from build123d import *

# Parameters (mm, degrees)
SKETCH1_R           = 1.450000001
SKETCH1_R_2         = 3.250000001
SKETCH1_R_3         = 1.5
SKETCH1_R_4         = 2.5
SKETCH1_R_5         = 1.375000001
BOSS_EXTRUDE2_DEPTH = 6.35


with BuildPart() as part:
    # Sketch1 → Boss-Extrude2 (new body)
    with BuildSketch(Plane.XY):
        with BuildLine():
            Line((-155.352886895, 10.211716756), (-51.913748531, 10.211716756))
            ThreePointArc((-51.913748531, 10.211716756), (-39.74822347, 6.086224622), (-32.601576204, -4.588283244))
            ThreePointArc((-32.601576204, -4.588283244), (53.610301025, -63.284580406), (124.587919611, 13.13479368))
            ThreePointArc((124.587919611, 13.13479368), (56.661218885, 95.304455124), (-32.601576204, 37.011716756))
            ThreePointArc((-32.601576204, 37.011716756), (-39.74822347, 26.33720889), (-51.913748531, 22.211716756))
            Line((-51.913748531, 22.211716756), (-155.352886895, 22.211716756))
            ThreePointArc((-155.352886895, 22.211716756), (-161.352886895, 16.211716756), (-155.352886895, 10.211716756))
        make_face()
        with Locations((-19.438766774, -20.788283242)):
            Circle(SKETCH1_R, mode=Mode.SUBTRACT)
        with Locations((-26.831398039, -2.940892579)):
            Circle(SKETCH1_R, mode=Mode.SUBTRACT)
        with Locations((-155.352886895, 16.211716756)):
            Circle(SKETCH1_R_2, mode=Mode.SUBTRACT)
        with Locations((-26.831398039, 35.364326096)):
            Circle(SKETCH1_R, mode=Mode.SUBTRACT)
        with Locations((-19.438766774, 53.211716759)):
            Circle(SKETCH1_R, mode=Mode.SUBTRACT)
        with Locations((-29.352886893, 16.211716758)):
            Circle(SKETCH1_R, mode=Mode.SUBTRACT)
        with Locations((44.647113106, 6.211716759)):
            Circle(SKETCH1_R_3, mode=Mode.SUBTRACT)
        with Locations((116.125624253, -2.940892579)):
            Circle(SKETCH1_R, mode=Mode.SUBTRACT)
        with Locations((108.732992988, -20.788283242)):
            Circle(SKETCH1_R, mode=Mode.SUBTRACT)
        with Locations((96.973014915, -36.114185049)):
            Circle(SKETCH1_R, mode=Mode.SUBTRACT)
        with Locations((81.647113106, -47.874163121)):
            Circle(SKETCH1_R, mode=Mode.SUBTRACT)
        with Locations((63.799722443, -55.266794386)):
            Circle(SKETCH1_R, mode=Mode.SUBTRACT)
        with Locations((44.647113106, -57.788283242)):
            Circle(SKETCH1_R, mode=Mode.SUBTRACT)
        with Locations((25.494503768, -55.266794386)):
            Circle(SKETCH1_R, mode=Mode.SUBTRACT)
        with Locations((7.647113108, -47.874163121)):
            Circle(SKETCH1_R, mode=Mode.SUBTRACT)
        with Locations((-7.678788702, -36.114185049)):
            Circle(SKETCH1_R, mode=Mode.SUBTRACT)
        with Locations((44.647113106, 16.211716756)):
            Circle(SKETCH1_R_4, mode=Mode.SUBTRACT)
        with Locations((-7.678788702, 68.537618566)):
            Circle(SKETCH1_R, mode=Mode.SUBTRACT)
        with Locations((7.647113108, 80.297596638)):
            Circle(SKETCH1_R, mode=Mode.SUBTRACT)
        with Locations((25.494503768, 87.690227903)):
            Circle(SKETCH1_R, mode=Mode.SUBTRACT)
        with Locations((44.647113106, 90.211716759)):
            Circle(SKETCH1_R, mode=Mode.SUBTRACT)
        with Locations((63.799722443, 87.690227903)):
            Circle(SKETCH1_R, mode=Mode.SUBTRACT)
        with Locations((81.647113106, 80.297596638)):
            Circle(SKETCH1_R, mode=Mode.SUBTRACT)
        with Locations((96.973014915, 68.537618566)):
            Circle(SKETCH1_R, mode=Mode.SUBTRACT)
        with Locations((108.732992988, 53.211716759)):
            Circle(SKETCH1_R, mode=Mode.SUBTRACT)
        with Locations((116.125624253, 35.364326096)):
            Circle(SKETCH1_R, mode=Mode.SUBTRACT)
        with Locations((44.647113106, 26.211716758)):
            Circle(SKETCH1_R_5, mode=Mode.SUBTRACT)
        with Locations((118.647113104, 16.211716758)):
            Circle(SKETCH1_R, mode=Mode.SUBTRACT)
        with BuildLine():
            Line((-4.014987137, 10.211716754), (22.197168785, 10.211716754))
            ThreePointArc((22.197168785, 10.211716754), (24.842920096, 9.454357441), (26.687157649, 7.411716754))
            ThreePointArc((26.687157649, 7.411716754), (44.647113107, -3.788283245), (62.607068564, 7.411716755))
            ThreePointArc((62.607068564, 7.411716755), (64.451306117, 9.454357442), (67.097057428, 10.211716755))
            Line((67.097057428, 10.211716755), (93.309213348, 10.211716755))
            ThreePointArc((93.309213348, 10.211716755), (105.842188723, 3.453350593), (107.081505871, -10.731679472))
            ThreePointArc((107.081505871, -10.731679472), (44.647113106, -51.788283245), (-17.787279658, -10.731679472))
            ThreePointArc((-17.787279658, -10.731679472), (-16.54796251, 3.453350591), (-4.014987137, 10.211716754))
        make_face(mode=Mode.SUBTRACT)
        with BuildLine():
            Line((93.309213348, 22.211716754), (67.097057429, 22.211716754))
            ThreePointArc((67.097057429, 22.211716754), (64.451306116, 22.969076068), (62.607068563, 25.011716756))
            ThreePointArc((62.607068563, 25.011716756), (44.647113106, 36.211716756), (26.68715765, 25.011716756))
            ThreePointArc((26.68715765, 25.011716756), (24.842920097, 22.969076069), (22.197168786, 22.211716756))
            Line((22.197168786, 22.211716756), (-4.014987136, 22.211716756))
            ThreePointArc((-4.014987136, 22.211716756), (-16.547962509, 28.970082919), (-17.787279657, 43.155112983))
            ThreePointArc((-17.787279657, 43.155112983), (44.647113107, 84.211716756), (107.08150587, 43.155112983))
            ThreePointArc((107.08150587, 43.155112983), (105.842188723, 28.970082917), (93.309213348, 22.211716754))
        make_face(mode=Mode.SUBTRACT)
    extrude(amount=BOSS_EXTRUDE2_DEPTH)


solid = part.part
Geometry: final body of the model. Coordinates: model frame, mm. A direction names the side the tool comes from. Give positions to 0.01 mm unless a question says otherwise; leave off trailing zeros. Write each loop counter-clockwise with the first axis right and the second up, starting at its lowest first coordinate (ties: lowest second). Pieces come first, ordered by that corner, then holes. Notation, with made-up numbers: (29.25, 25) - (39.25, 25) arc R27 cw to (39.25, 57) - close; hole circle Ø5 at (64.5, 54.5). An arc over 180 degrees is marked (long way). Return JSON: item names as keys, results as strings. Group by question number.
1) First-contact query: P1, Ø4.5, axis at x = -26.83, y = -2.94, coming from the +Z side; P2, Ø1.9, axis at x = -86.5, z = 3.5, coming from the +Y side. Flat tips, straight axial feed; report the tip coordinate or a pass-through.
2) Section C-C on z = 1.5. State how many separate pieces and enclosed holes the cut face has, plus the area to 3 significant figures.
3) Set-up query: faces 4 (the cylindrical face through (44.335, -3.786, 3.131)), 5 (the flat face through (-103, 22.212, 3)), 6 (the flat face through (-104, 10.212, 3)), 7 (the flat face through (23, 11, 6.35)). Return all of +Z, -Z, +X, -X, +Y, -Y with unobstructed straight access to the full face (end or side cutting, diameter ignored); none if empty.
4) Section A-A on x = 15. Return the cut outline in (y, z).
5) Mould query, pull axis Y, two halves, no side actions, for faces 1 (the cylindrical face through (-39.9, 6.2, 3.1)), 2 (the cylindrical face through (-39.6, 26.45, 3.13)), 3 (the flat face through (80, 10.212, 3)). Classes: released by +Y, released by -Y, zero draft, split by the parting line, or undercut.
6) Section D-D on x = -84.5. Return the cut outline in (y, z), plus the area to 3 significant figures.
7) Line query: line 1 (X direction, y = 79, z = 0.5); line 2 (Y direction, x = 55, z = 4.5); line 3 (X direction, y = 3, z = 1.25). Output: solid intervals per line, ascending.
8) Section B-B on y = 31. Return the cut outline in (x, z), plus the area to 3 significant figures.
Filled in:
{
 "1": {"P1": "stops at z = 6.35", "P2": "stops at y = 22.21"},
 "2": {"separate pieces": "1", "enclosed holes": "30", "area": "9,750 mm^2"},
 "3": {"face 4": "+Z, -Z", "face 5": "+Z, -Z, -X, +Y", "face 6": "+Z, -Z, -X, -Y", "face 7": "+Z, +X, -X, +Y, -Y"},
 "4": {"outline": "(-58.09, 0) - (-44.99, 0) - (-44.99, 6.35) - (-58.09, 6.35) - close; (10.21, 0) - (22.21, 0) - (22.21, 6.35) - (10.21, 6.35) - close; (77.41, 0) - (90.52, 0) - (90.52, 6.35) - (77.41, 6.35) - close"},
 "5": {"face 1": "released by -Y", "face 2": "released by +Y", "face 3": "undercut"},
 "6": {"outline": "(10.21, 0) - (22.21, 0) - (22.21, 6.35) - (10.21, 6.35) - close", "area": "76.2 mm^2"},
 "7": {"line 1": "x = -4.93 to 7, 8.29 to 18.54, 70.76 to 81, 82.29 to 94.22", "line 2": "y = -63.12 to -51, -0.9 to 33.32, 83.42 to 95.54", "line 3": "x = -36.54 to -16.83, 29.63 to 59.66, 106.13 to 123.55"},
 "8": {"outline": "(-35.35, 0) - (-17.67, 0) - (-17.67, 6.35) - (-35.35, 6.35) - close; (31.18, 0) - (58.11, 0) - (58.11, 6.35) - (31.18, 6.35) - close; (106.96, 0) - (123.27, 0) - (123.27, 6.35) - (106.96, 6.35) - close", "area": "387 mm^2"}
}
